For this review, take the finished solid that the model builds, in its own axes (mm). Face numbers are marked on the shaded views. A direction names the side the tool comes from. Round coordinates to 2 decimals unless told otherwise and drop trailing zeros. Write each loop counter-clockwise with the first axis right and the second up, starting at its lowest first coordinate (ties: lowest second). Pieces come first, ordered by that corner, then holes. Notation, with made-up numbers: M 73,53.25 L 82,53.25 A13 cw 82,69.25 Z; hole C 56,43.25 d1. An arc over 180 degrees is marked long. Write each question's results on one line, items separated by ' | '. Start each with the question number.
Autodesk Inventor part; units mm, degrees
ref_plane "YZ Plane" through (0, 0, 0) normal (1, 0, 0) x (0, 1, 0)
ref_plane "XZ Plane" through (0, 0, 0) normal (0, 1, 0) x (-1, 0, 0)
ref_plane "XY Plane" through (0, 0, 0) normal (0, 0, 1) x (1, 0, 0)
sketch "Sketch2" plane through (0, 0, 0) normal (0, 0, 1) x (1, 0, 0)
  line L0 (0, 0) -> (19.05, 0)
  line L1 (19.05, 0) -> (19.05, 6.35)
  line L2 (12.7, 12.7) -> (0, 12.7)
  line L3 (0, 12.7) -> (0, 0)
  arc A0 (19.05, 6.35) -> (12.7, 12.7) centre (12.7, 6.35) ccw
  line L4 (19.05, 6.35) -> (12.7, 6.35)
  line L5 (12.7, 6.35) -> (12.7, 0)
  line L6 (4.7625, 0) -> (4.7625, -3.6847)
  line L7 (4.7625, -3.6847) -> (6.35, -3.6847)
  line L8 (6.35, -3.6847) -> (6.35, 0)
  dimension "d8" = 6.35
  dimension "d9" = 12.7
  dimension "d10" = 19.05
  dimension "d11" = 7.9375
  dimension "d12" = 1.5875
revolve "Revolution1" add sketch "Sketch2" angle 360 about axis through (0, 12.7, 0) along (0, -1, 0) contours L3 L2 A0 L4 L5 L0 | L0 L8 L7 L6
sketch "Sketch3" plane through (0, 12.7, 0) normal (0, 1, 0) x (1, 0, 0)
  circle A0 centre (0, 0) radius 4.7625
  dimension "d14" = 9.525
extrude "Extrusion1" cut sketch "Sketch3" against normal through all
sketch "Sketch4" plane through (0, 12.7, 0) normal (0, 1, 0) x (1, 0, 0)
  circle A0 centre (0, 0) radius 12.7
  line L0 (-12.7, 0) -> (0, 12.7)
  line L1 (12.7, 0) -> (0, 12.7)
  line L2 (12.7, 0) -> (0, -12.7)
  line L3 (-12.7, 0) -> (0, -12.7)
extrude "Extrusion2" cut sketch "Sketch4" against normal blind 1.5875 contours L2 L3 L0 L1
equation "\"d15\" = d14"
properties part number "sleeve_support"
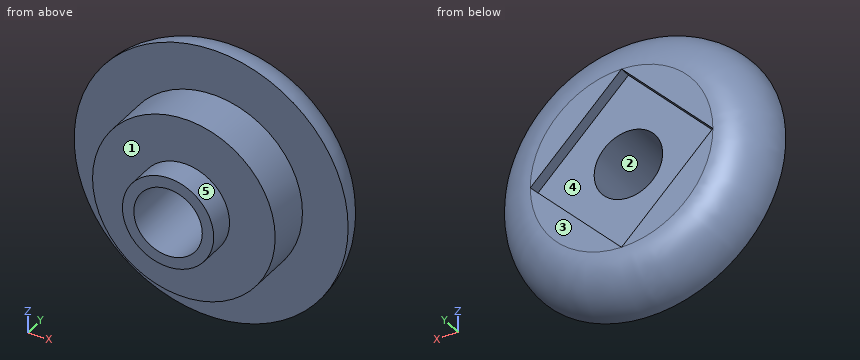
Item 1: For the marked faces 1 and 2, list the 3-axis set-ups (+Z, -Z, +X, -X, +Y, -Y) from which the entire face can be reached by the end or side of a thin tool; tool diameter is ignored.
Item 2: For probe 1 along Z at (x, y) = (0, 0.75); probe 2 along Y at (x, z) = (3.5, 10.5); probe 3 along X at (y, z) = (2, 11), list the stretches that pass through material, from the lowest coordinate up.
Item 3: Mouldability with a two-part tool opening along X and no side actions: class the marked faces 3, 4 and 5 as pulls with the +X half, pulls with the -X half, needs draft (parallel to the pull), parting line crosses it, or undercut.
Item 4: We need section A-A on y = 3.5. State the section outline as (x, z) points (1 decimal), then the cut area to 3 significant figures.
Item 5: Insertion check: P1, Ø1.5, axis at x = -4.5, z = -9, coming from the -Y side; P2, Ø3, axis at y = 1.5, z = -4.5, coming from the +X side; P3, Ø2, axis at y = 6, z = -13.5, coming from the -X side. Each pin has a flat end and moves straight along its axis. Give the tip position at first contact, or say it passes through.
Numbers:
1) face 1: -Y | face 2: +Y, -Y
2) probe 1: z = -12.7 to -4.76, 4.76 to 12.7 | probe 2: y = 0 to 12.7 | probe 3: x = -6.35 to 6.35
3) face 3: needs draft | face 4: undercut | face 5: parting line crosses it
4) outline: C 0,0 d25.4; hole C 0,0 d9.5 | area: 435 mm^2
5) P1: stops at y = 0 | P2: stops at x = 12.34 | P3: stops at x = -14.32
